```python
from build123d import *

# Parameters (mm, degrees)
F0_W         = 18
F0_H         = 7
F1_DEPTH     = 5
F2_W         = 21
F2_H         = 4
F3_DEPTH     = 4
F4_T4_DEPTH  = 37.431305486
F4_T9_DEPTH  = 33.931305486
F4_T15_DEPTH = 33.931305486
F4_T21_DEPTH = 37.431305486
F5_R         = 0.5
F6_T1_DEPTH  = 2.8169048105
F6_T3_DEPTH  = 2.8169048105
F6_T5_DEPTH  = 0.2169048105
F6_T7_DEPTH  = 4.0985711369
F6_T9_DEPTH  = 0.2169048105
F6_T11_DEPTH = 4.0985711369
F6_S15_W     = 0.5
F6_S15_H     = 0.5
F6_T16_DEPTH = 0.5
F6_S21_W     = 0.5
F6_S21_H     = 0.5
F6_T22_DEPTH = 0.5
F6_S27_W     = 0.5
F6_S27_H     = 0.5
F6_T28_DEPTH = 0.5
F6_S33_W     = 0.5
F6_S33_H     = 0.5
F6_T34_DEPTH = 0.5
F6_T38_ANGLE = 59.0362434679
F6_T40_ANGLE = 59.0362434679
F6_T42_ANGLE = 59.0362434679
F6_T44_ANGLE = 59.0362434679


# Not quite as in the source:
# - a fillet or chamfer that OpenCascade refuses, or shapes differently, is made with other operations: its cross-section is extruded or revolved along the edge and cut away or added


with BuildPart() as f1:
    # F0 (on Top) → F1 (new body)
    with BuildSketch(Plane.XY):
        Polygon((-41.0881050097, 20.8523701802), (-48.0881050097, 20.8523701802), (-48.0881050097, -7.6476298198), (-41.0881050097, -7.6476298198), (-41.0881050097, 13.8523701802), align=None)
        with Locations((-32.0881050097, 17.3523701802)):
            Rectangle(F0_W, F0_H)
    extrude(amount=F1_DEPTH)

    # F2 (on face) → F3 (join)
    with BuildSketch(Plane.XY.offset(5)):
        Polygon((-44.0881050097, 20.8523701802), (-48.0881050097, 20.8523701802), (-48.0881050097, -7.6476298198), (-44.0881050097, -7.6476298198), (-44.0881050097, 16.8523701802), align=None)
        with Locations((-33.5881050097, 18.8523701802)):
            Rectangle(F2_W, F2_H)
    extrude(amount=F3_DEPTH)

    # F4: chamfer of 5 x 3 on 2 edges, made by hand


with BuildPart() as f4_tool2:
    # F4_s3 → F4_t4 (new body)
    with BuildSketch(Plane.XZ.offset(20.5789353058)):
        Polygon((-44.0881050097, 4), (-47.0881050097, 9), (-44.0881050097, 9), align=None)
    extrude(amount=-F4_T4_DEPTH)

    split(bisect_by=Plane.XY.offset(5), keep=Keep.TOP)


with BuildPart() as f1_1:
    add(f1.part)

    # F4_t1: cut F4_tool2
    add(f4_tool2.part, mode=Mode.SUBTRACT)


with BuildPart() as f4_tool7:
    # F4_s8 → F4_t9 (new body)
    with BuildSketch(Plane.YZ.offset(-44.0881050097)):
        Polygon((16.8523701802, 4), (19.8523701802, 9), (16.8523701802, 9), align=None)
    extrude(amount=F4_T9_DEPTH)

    split(bisect_by=Plane.XY.offset(5), keep=Keep.TOP)


with BuildPart() as f1_2:
    add(f1_1.part)

    # F4_t6: cut F4_tool7
    add(f4_tool7.part, mode=Mode.SUBTRACT)


with BuildPart() as f4_tool13:
    # F4_s14 → F4_t15 (new body)
    with BuildSketch(Plane.YZ.offset(-57.0194104957)):
        Polygon((16.8523701802, 4), (19.8523701802, 9), (16.8523701802, 9), align=None)
    extrude(amount=F4_T15_DEPTH)

    split(bisect_by=Plane.YZ.offset(-48.0881050097), keep=Keep.TOP)

    split(bisect_by=Plane.YZ.offset(-44.0881050097), keep=Keep.BOTTOM)

    split(bisect_by=Plane.XY.offset(5), keep=Keep.TOP)


with BuildPart() as f4_tool19:
    # F4_s20 → F4_t21 (new body)
    with BuildSketch(Plane.XZ.offset(7.6476298198)):
        Polygon((-44.0881050097, 4), (-47.0881050097, 9), (-44.0881050097, 9), align=None)
    extrude(amount=-F4_T21_DEPTH)

    split(bisect_by=Plane.XZ.offset(-16.8523701802), keep=Keep.BOTTOM)

    split(bisect_by=Plane.XY.offset(5), keep=Keep.TOP)

    split(bisect_by=Plane.XZ.offset(-20.8523701802), keep=Keep.TOP)


with BuildPart() as f4_tool13_1:
    add(f4_tool13.part)

    # F4_t25: intersect F4_tool19
    add(f4_tool19.part, mode=Mode.INTERSECT)


with BuildPart() as f1_3:
    add(f1_2.part)

    # F4_t11: cut F4_tool13
    add(f4_tool13_1.part, mode=Mode.SUBTRACT)

    # F5
    f5_edges = [f1_3.edges().sort_by_distance(p)[0] for p in [
        (-48.088105, -7.64763, 4.5),
        (-41.088105, -7.64763, 2.5),
        (-41.088105, 13.85237, 2.5),
        (-23.088105, 13.85237, 2.5),
        (-23.088105, 20.85237, 4.5),
        (-35.588105, 20.85237, 9),
        (-35.088105, 19.85237, 9),
        (-47.088105, 6.10237, 9),
        (-45.888105, 18.65237, 7),
        (-33.888105, 17.45237, 5),
        (-44.688105, 4.90237, 5),
        (-41.088105, 3.10237, 5),
        (-32.088105, 13.85237, 5),
        (-48.088105, 6.60237, 9),
        (-48.088105, 20.85237, 4.5),
    ]]
    fillet(f5_edges, radius=F5_R)

    # F6: fillet of radius 0.5 on 10 edges, made by hand

    # F6_s2 → F6_t1 (cut)
    with BuildSketch(Plane.YZ.offset(-44.4050098202)):
        with BuildLine():
            ThreePointArc((-7.6476298198, 4.5), (-7.5011832104, 4.8535533906), (-7.1476298198, 5))
            Line((-7.1476298198, 5), (-7.6476298198, 5))
            Line((-7.6476298198, 5), (-7.6476298198, 4.5))
        make_face()
    extrude(amount=F6_T1_DEPTH, mode=Mode.SUBTRACT)

    # F6_s4 → F6_t3 (cut)
    with BuildSketch(Plane.XZ.offset(-17.1692749907)):
        with BuildLine():
            ThreePointArc((-23.0881050097, 4.5), (-23.2345516191, 4.8535533906), (-23.5881050097, 5))
            Line((-23.5881050097, 5), (-23.0881050097, 5))
            Line((-23.0881050097, 5), (-23.0881050097, 4.5))
        make_face()
    extrude(amount=F6_T3_DEPTH, mode=Mode.SUBTRACT)

    # F6_s6 → F6_t5 (cut)
    with BuildSketch(Plane.YZ.offset(-47.5881050097)):
        with BuildLine():
            ThreePointArc((-7.6476298198, 8.5), (-7.5011832104, 8.8535533906), (-7.1476298198, 9))
            Line((-7.1476298198, 9), (-7.6476298198, 9))
            Line((-7.6476298198, 9), (-7.6476298198, 8.5))
        make_face()
    extrude(amount=F6_T5_DEPTH, mode=Mode.SUBTRACT)

    # F6_s8 → F6_t7 (cut)
    with BuildSketch(Plane(origin=(-16.2894353468, 0, 27.1490589114), x_dir=(0, 1, 0), z_dir=(0.5144957554, 0, -0.8574929257))):
        with BuildLine():
            ThreePointArc((-7.6476298198, -36.2472551322), (-7.5011832104, -35.8937017416), (-7.1476298198, -35.7472551322))
            Line((-7.1476298198, -35.7472551322), (-7.6476298198, -35.7472551322))
            Line((-7.6476298198, -35.7472551322), (-7.6476298198, -36.2472551322))
        make_face()
    extrude(amount=F6_T7_DEPTH, mode=Mode.SUBTRACT)

    # F6_s10 → F6_t9 (cut)
    with BuildSketch(Plane.XZ.offset(-20.3523701802)):
        with BuildLine():
            ThreePointArc((-23.0881050097, 8.5), (-23.2345516191, 8.8535533906), (-23.5881050097, 9))
            Line((-23.5881050097, 9), (-23.0881050097, 9))
            Line((-23.0881050097, 9), (-23.0881050097, 8.5))
        make_face()
    extrude(amount=F6_T9_DEPTH, mode=Mode.SUBTRACT)

    # F6_s12 → F6_t11 (cut)
    with BuildSketch(Plane(origin=(0, 6.971278674, 11.61879779), x_dir=(1, 0, 0), z_dir=(0, 0.5144957554, 0.8574929257))):
        with BuildLine():
            ThreePointArc((-23.0881050097, 12.8928051893), (-23.2345516191, 12.5392517987), (-23.5881050097, 12.3928051893))
            Line((-23.5881050097, 12.3928051893), (-23.0881050097, 12.3928051893))
            Line((-23.0881050097, 12.3928051893), (-23.0881050097, 12.8928051893))
        make_face()
    extrude(amount=F6_T11_DEPTH, mode=Mode.SUBTRACT)


with BuildPart() as f6_tool14:
    # F6_s15 → F6_t16 (new body)
    with BuildSketch(Plane.YZ.offset(-23.5881050097)):
        with Locations((20.6023701802, 8.75)):
            Rectangle(F6_S15_W, F6_S15_H)
    extrude(amount=F6_T16_DEPTH)

    # F6_s17 → F6_t18 (revolve, cut)
    with BuildSketch(Plane(origin=(-23.5881050097, 20.3523701802, 8.5), x_dir=(0, -0.7071067812, -0.7071067812), z_dir=(0, -0.7071067812, 0.7071067812))):
        with BuildLine():
            ThreePointArc((0, -0.5), (0.5, 0), (0, 0.5))
            Line((0, 0.5), (0, -0.5))
        make_face()
    revolve(axis=Axis((-23.5881050097, 20.3523701802, 8.5), (1, 0, 0)), mode=Mode.SUBTRACT)


with BuildPart() as f1_4:
    add(f1_3.part)

    # F6_t13: cut F6_tool14
    add(f6_tool14.part, mode=Mode.SUBTRACT)


with BuildPart() as f6_tool20:
    # F6_s21 → F6_t22 (new body)
    with BuildSketch(Plane.XZ.offset(7.1476298198)):
        with Locations((-47.8381050097, 8.75)):
            Rectangle(F6_S21_W, F6_S21_H)
    extrude(amount=F6_T22_DEPTH)

    # F6_s23 → F6_t24 (revolve, cut)
    with BuildSketch(Plane(origin=(-47.5881050097, -7.1476298198, 8.5), x_dir=(0.7071067812, 0, -0.7071067812), z_dir=(-0.7071067812, 0, -0.7071067812))):
        with BuildLine():
            ThreePointArc((0, -0.5), (0.5, 0), (0, 0.5))
            Line((0, 0.5), (0, -0.5))
        make_face()
    revolve(axis=Axis((-47.5881050097, -7.1476298198, 8.5), (0, -1, 0)), mode=Mode.SUBTRACT)


with BuildPart() as f1_5:
    add(f1_4.part)

    # F6_t19: cut F6_tool20
    add(f6_tool20.part, mode=Mode.SUBTRACT)


with BuildPart() as f6_tool26:
    # F6_s27 → F6_t28 (new body)
    with BuildSketch(Plane.YZ.offset(-23.5881050097)):
        with Locations((14.1023701802, 4.75)):
            Rectangle(F6_S27_W, F6_S27_H)
    extrude(amount=F6_T28_DEPTH)

    # F6_s29 → F6_t30 (revolve, cut)
    with BuildSketch(Plane(origin=(-23.5881050097, 14.3523701802, 4.5), x_dir=(0, 0.7071067812, -0.7071067812), z_dir=(0, -0.7071067812, -0.7071067812))):
        with BuildLine():
            ThreePointArc((0, -0.5), (0.5, 0), (0, 0.5))
            Line((0, 0.5), (0, -0.5))
        make_face()
    revolve(axis=Axis((-23.5881050097, 14.3523701802, 4.5), (1, 0, 0)), mode=Mode.SUBTRACT)


with BuildPart() as f1_6:
    add(f1_5.part)

    # F6_t25: cut F6_tool26
    add(f6_tool26.part, mode=Mode.SUBTRACT)


with BuildPart() as f6_tool32:
    # F6_s33 → F6_t34 (new body)
    with BuildSketch(Plane.XZ.offset(7.1476298198)):
        with Locations((-41.3381050097, 4.75)):
            Rectangle(F6_S33_W, F6_S33_H)
    extrude(amount=F6_T34_DEPTH)

    # F6_s35 → F6_t36 (revolve, cut)
    with BuildSketch(Plane(origin=(-41.5881050097, -7.1476298198, 4.5), x_dir=(-0.7071067812, 0, -0.7071067812), z_dir=(-0.7071067812, 0, 0.7071067812))):
        with BuildLine():
            ThreePointArc((0, -0.5), (0.5, 0), (0, 0.5))
            Line((0, 0.5), (0, -0.5))
        make_face()
    revolve(axis=Axis((-41.5881050097, -7.1476298198, 4.5), (0, -1, 0)), mode=Mode.SUBTRACT)


with BuildPart() as f1_7:
    add(f1_6.part)

    # F6_t31: cut F6_tool32
    add(f6_tool32.part, mode=Mode.SUBTRACT)

    # F6_s37 → F6_t38 (revolve, cut)
    with BuildSketch(Plane(origin=(-16.2894353468, 0, 27.1490589114), x_dir=(0, 1, 0), z_dir=(0.5144957554, 0, -0.8574929257))):
        with BuildLine():
            ThreePointArc((-7.6476298198, -36.2472551322), (-7.5011832104, -35.8937017416), (-7.1476298198, -35.7472551322))
            Line((-7.1476298198, -35.7472551322), (-7.6476298198, -35.7472551322))
            Line((-7.6476298198, -35.7472551322), (-7.6476298198, -36.2472551322))
        make_face()
    revolve(axis=Axis((-47.3712001992, -7.6476298198, 8.5), (0, -1, 0)), revolution_arc=F6_T38_ANGLE, mode=Mode.SUBTRACT)

    # F6_s39 → F6_t40 (revolve, cut)
    with BuildSketch(Plane(origin=(-14.1807378936, 0, 23.634563156), x_dir=(0, 1, 0), z_dir=(-0.5144957554, 0, 0.8574929257))):
        with BuildLine():
            ThreePointArc((-7.6476298198, 36.2472551322), (-7.5011832104, 35.8937017416), (-7.1476298198, 35.7472551322))
            Line((-7.1476298198, 35.7472551322), (-7.6476298198, 35.7472551322))
            Line((-7.6476298198, 35.7472551322), (-7.6476298198, 36.2472551322))
        make_face()
    revolve(axis=Axis((-44.4050098202, -7.6476298198, 5.5), (0, -1, 0)), revolution_arc=F6_T40_ANGLE, mode=Mode.SUBTRACT)

    # F6_s41 → F6_t42 (revolve, cut)
    with BuildSketch(Plane(origin=(0, 6.971278674, 11.61879779), x_dir=(1, 0, 0), z_dir=(0, 0.5144957554, 0.8574929257))):
        with BuildLine():
            ThreePointArc((-23.0881050097, 12.8928051893), (-23.2345516191, 12.5392517987), (-23.5881050097, 12.3928051893))
            Line((-23.5881050097, 12.3928051893), (-23.0881050097, 12.3928051893))
            Line((-23.0881050097, 12.3928051893), (-23.0881050097, 12.8928051893))
        make_face()
    revolve(axis=Axis((-23.0881050097, 17.1692749907, 5.5), (-1, 0, 0)), revolution_arc=F6_T42_ANGLE, mode=Mode.SUBTRACT)

    # F6_s43 → F6_t44 (revolve, cut)
    with BuildSketch(Plane(origin=(0, 9.0799761273, 15.1332935454), x_dir=(1, 0, 0), z_dir=(0, -0.5144957554, -0.8574929257))):
        with BuildLine():
            ThreePointArc((-23.0881050097, -12.8928051893), (-23.2345516191, -12.5392517987), (-23.5881050097, -12.3928051893))
            Line((-23.5881050097, -12.3928051893), (-23.0881050097, -12.3928051893))
            Line((-23.0881050097, -12.3928051893), (-23.0881050097, -12.8928051893))
        make_face()
    revolve(axis=Axis((-23.0881050097, 20.1354653697, 8.5), (-1, 0, 0)), revolution_arc=F6_T44_ANGLE, mode=Mode.SUBTRACT)


solid = f1_7.part
```
Can you work these out from the model? Positions are in its coordinate system, mm. A direction names the side the tool comes from. Coordinates: 2 decimals unless noted, no trailing zeros. Order: outer loops, then holes, each group sorted by start corner. A loop starts at its lowest first (then second) coordinate and runs counter-clockwise, first axis right, second up.
1. If we section it at A-A (z = 3.75): Please give me the cut outline in (x, y).
2. For faces 1 (the face through (-42, 9, 5)), 2 (the face through (-41.088, 3, 2)), 3 (the face through (-23.088, 18, 3)), which set-ups out of +Z, -Z, +X, -X, +Y, -Y let a thin tool reach every point of the face, with its end or its side?
3. I'm going to push flat-ended pins straight in: pin 1 (1.3 mm diameter, centred on x = -35, z = 2.5, fed in from -Y); pin 2 (3.5 mm diameter, centred on y = -1.5, z = 2, fed in from +X); pin 3 (1.5 mm diameter, centred on x = -33.5, y = 12, fed in from +Z); pin 4 (6 mm diameter, centred on x = -40.5, y = 6.5, fed in from -Z). Where does each tip first touch, or does it pass through?
4. If we section it at C-C (x = -25.5): Please give me the cut outline in (y, z), then the cut area to 3 significant figures.
5. If we section it at B-B (y = 15): Please give me the cut outline in (x, z) (3 decimals).
6. I need wall thicknesses on line 1 (Y direction, x = -23.75, z = 2.25); line 2 (Z direction, x = -28, y = 15); line 3 (X direction, y = 7, z = 3.5). Which ranges of each line are inside material? Lowest first, please.
Entries:
1. outline: (-48.09, -7.15) arc R0.5 ccw to (-47.59, -7.65) - (-41.59, -7.65) arc R0.5 ccw to (-41.09, -7.15) - (-41.09, 13.35) arc R0.5 cw to (-40.59, 13.85) - (-23.59, 13.85) arc R0.5 ccw to (-23.09, 14.35) - (-23.09, 20.35) arc R0.5 ccw to (-23.59, 20.85) - (-47.59, 20.85) arc R0.5 ccw to (-48.09, 20.35) - close
2. face 1: +Z, +X, -Y
2. face 2: +Z, -Z, +X, -Y
2. face 3: +Z, -Z, +X, +Y, -Y
3. pin 1: stops at y = 13.85
3. pin 2: stops at x = -41.09
3. pin 3: passes through
3. pin 4: stops at z = 0
4. outline: (13.85, 0) - (20.85, 0) - (20.85, 8.5) arc R0.5 ccw to (20.35, 9) - (20.14, 9) arc R0.5 ccw to (19.71, 8.76) - (17.6, 5.24) arc R0.5 cw to (17.17, 5) - (14.35, 5) arc R0.5 ccw to (13.85, 4.5) - close
4. area: 43.7 mm2
5. outline: (-48.088, 0) - (-23.088, 0) - (-23.088, 4.5) arc R0.5 ccw to (-23.588, 5) - (-44.405, 5) arc R0.5 cw to (-44.834, 5.243) - (-46.942, 8.757) arc R0.5 ccw to (-47.371, 9) - (-47.588, 9) arc R0.5 ccw to (-48.088, 8.5) - close
6. line 1: y = 13.85 to 20.85
6. line 2: z = 0 to 5
6. line 3: x = -48.09 to -41.09
